The listing builds one solid part. Answer for the finished solid, in the listing's coordinates (mm). A direction names the side the tool comes from. Give positions to 0.01 mm unless a question says otherwise; leave off trailing zeros. Order: outer loops, then holes, each group sorted by start corner. A loop starts at its lowest first (then second) coordinate and runs counter-clockwise, first axis right, second up.
```python
from build123d import *

# Parameters (mm, degrees)
F0_R     = 9.525
F0_R_2   = 5.08
F0_R_3   = 6.35
F0_R_4   = 7.668055
F1_DEPTH = 6.35
F2_DEPTH = 3.175
F3_DEPTH = 12.7


with BuildPart() as f1:
    # F0 (on Front) → F1 (new body, symmetric)
    with BuildSketch(Plane.XZ):
        with BuildLine():
            ThreePointArc((-47.831061, 12.261839), (-40.825144, 16.749128), (-38.1, 24.609932))
            ThreePointArc((-38.1, 24.609932), (-38.532742, 27.896934), (-39.801477, 30.959932))
            ThreePointArc((-39.801477, 30.959932), (-44.45, 35.608455), (-50.8, 37.309932))
            ThreePointArc((-50.8, 37.309932), (-62.469497, 29.621203), (-60.009293, 15.864709))
            ThreePointArc((-60.009293, 15.864709), (-54.40287, 12.4317), (-47.831061, 12.261839))
        make_face()
        with Locations((-50.8, 24.609932)):
            Circle(F0_R, mode=Mode.SUBTRACT)
        with BuildLine():
            ThreePointArc((-50.8, 37.309932), (-44.45, 35.608455), (-39.801477, 30.959932))
            Line((-39.801477, 30.959932), (-6.35, 30.959932))
            ThreePointArc((-6.35, 30.959932), (-4.490128, 35.45006), (0, 37.309932))
            Line((0, 37.309932), (-50.8, 37.309932))
        make_face()
        with BuildLine():
            ThreePointArc((0, 37.309932), (-4.490128, 35.45006), (-6.35, 30.959932))
            ThreePointArc((-6.35, 30.959932), (0, 24.609932), (6.35, 30.959932))
            ThreePointArc((6.35, 30.959932), (4.490128, 35.45006), (0, 37.309932))
        make_face()
        with Locations((0, 30.959932)):
            Circle(F0_R_2, mode=Mode.SUBTRACT)
        with BuildLine():
            Line((50.8, 37.309932), (0, 37.309932))
            ThreePointArc((0, 37.309932), (4.490128, 35.45006), (6.35, 30.959932))
            Line((6.35, 30.959932), (39.801477, 30.959932))
            ThreePointArc((39.801477, 30.959932), (44.45, 35.608455), (50.8, 37.309932))
        make_face()
        with BuildLine():
            ThreePointArc((63.5, 24.609932), (59.780256, 33.590188), (50.8, 37.309932))
            ThreePointArc((50.8, 37.309932), (44.45, 35.608455), (39.801477, 30.959932))
            ThreePointArc((39.801477, 30.959932), (39.130503, 19.598661), (47.831061, 12.261839))
            ThreePointArc((47.831061, 12.261839), (54.40287, 12.4317), (60.009293, 15.864709))
            ThreePointArc((60.009293, 15.864709), (62.595084, 19.901855), (63.5, 24.609932))
        make_face()
        with Locations((50.8, 24.609932)):
            Circle(F0_R_3, mode=Mode.SUBTRACT)
        with BuildLine():
            Line((47.831061, 12.261839), (14.819522, -22.501475))
            ThreePointArc((14.819522, -22.501475), (15.029956, -23.943953), (15.10032, -25.4))
            ThreePointArc((15.10032, -25.4), (14.024374, -30.997911), (10.949864, -35.798084))
            Line((10.949864, -35.798084), (60.009293, 15.864709))
            ThreePointArc((60.009293, 15.864709), (54.40287, 12.4317), (47.831061, 12.261839))
        make_face()
        with BuildLine():
            ThreePointArc((14.819522, -22.501475), (0, -10.29968), (-14.819522, -22.501475))
            ThreePointArc((-14.819522, -22.501475), (-14.498802, -29.619527), (-10.949864, -35.798084))
            ThreePointArc((-10.949864, -35.798084), (0, -40.50032), (10.949864, -35.798084))
            ThreePointArc((10.949864, -35.798084), (14.024374, -30.997911), (15.10032, -25.4))
            ThreePointArc((15.10032, -25.4), (15.029956, -23.943953), (14.819522, -22.501475))
        make_face()
        with Locations((0, -25.4)):
            Circle(F0_R_4, mode=Mode.SUBTRACT)
        with BuildLine():
            Line((-14.819522, -22.501475), (-47.831061, 12.261839))
            ThreePointArc((-47.831061, 12.261839), (-54.40287, 12.4317), (-60.009293, 15.864709))
            Line((-60.009293, 15.864709), (-10.949864, -35.798084))
            ThreePointArc((-10.949864, -35.798084), (-14.498802, -29.619527), (-14.819522, -22.501475))
        make_face()
    extrude(amount=F1_DEPTH, both=True)

    # F0 (on Front) → F2 (join, symmetric)
    with BuildSketch(Plane.XZ):
        with BuildLine():
            ThreePointArc((-39.801477, 30.959932), (-38.532742, 27.896934), (-38.1, 24.609932))
            ThreePointArc((-38.1, 24.609932), (-40.825144, 16.749128), (-47.831061, 12.261839))
            Line((-47.831061, 12.261839), (-14.819522, -22.501475))
            ThreePointArc((-14.819522, -22.501475), (0, -10.29968), (14.819522, -22.501475))
            Line((14.819522, -22.501475), (47.831061, 12.261839))
            ThreePointArc((47.831061, 12.261839), (39.130503, 19.598661), (39.801477, 30.959932))
            Line((39.801477, 30.959932), (6.35, 30.959932))
            ThreePointArc((6.35, 30.959932), (0, 24.609932), (-6.35, 30.959932))
            Line((-6.35, 30.959932), (-39.801477, 30.959932))
        make_face()
    extrude(amount=F2_DEPTH, both=True)

    # F0 (on Front) → F3 (join, symmetric)
    with BuildSketch(Plane.XZ):
        with BuildLine():
            ThreePointArc((63.5, 24.609932), (59.780256, 33.590188), (50.8, 37.309932))
            ThreePointArc((50.8, 37.309932), (44.45, 35.608455), (39.801477, 30.959932))
            ThreePointArc((39.801477, 30.959932), (39.130503, 19.598661), (47.831061, 12.261839))
            ThreePointArc((47.831061, 12.261839), (54.40287, 12.4317), (60.009293, 15.864709))
            ThreePointArc((60.009293, 15.864709), (62.595084, 19.901855), (63.5, 24.609932))
        make_face()
        with Locations((50.8, 24.609932)):
            Circle(F0_R_3, mode=Mode.SUBTRACT)
    extrude(amount=F3_DEPTH, both=True)


solid = f1.part
```
1) For a pull along Z with two mould halves and no side action, classify faces 1 (the cylindrical face through (-46.4, 0.09, 16.16)), 2 (the flat face through (45, 12.7, 28)), 3 (the cylindrical face through (-62.386, -0.089, 29.811)) as +Z half, -Z half, draft (parallel to the pull), parting line (faces both ways), or undercut.
Geometry says:
face 1: undercut
face 2: draft
face 3: parting line
2) Find section C-C (z = -25.4). Write down the section's boundary in (x, y), then the cut area to 3 significant figures.
Geometry says:
outline: (-20.82, -6.35) - (-7.67, -6.35) - (-7.67, 6.35) - (-20.82, 6.35) - close; (7.67, -6.35) - (20.82, -6.35) - (20.82, 6.35) - (7.67, 6.35) - close
area: 334 mm2
3) Find section B-B (z = 21). Write down the section's boundary in (x, y) (3 decimals).
Geometry says:
outline: (-62.976, -6.35) - (-59.614, -6.35) - (-59.614, 6.35) - (-62.976, 6.35) - close; (-41.986, -6.35) - (-38.624, -6.35) - (-38.624, -3.175) - (38.624, -3.175) - (38.624, -12.7) - (45.576, -12.7) - (45.576, 12.7) - (38.624, 12.7) - (38.624, 3.175) - (-38.624, 3.175) - (-38.624, 6.35) - (-41.986, 6.35) - close; (56.024, -12.7) - (62.976, -12.7) - (62.976, 12.7) - (56.024, 12.7) - close
4) Find section A-A (x = 0). Write down the section's boundary in (y, z) (3 decimals).
Geometry says:
outline: (-6.35, -40.5) - (6.35, -40.5) - (6.35, -33.068) - (-6.35, -33.068) - close; (-6.35, -17.732) - (6.35, -17.732) - (6.35, -10.3) - (3.175, -10.3) - (3.175, 24.61) - (6.35, 24.61) - (6.35, 25.88) - (-6.35, 25.88) - (-6.35, 24.61) - (-3.175, 24.61) - (-3.175, -10.3) - (-6.35, -10.3) - close; (-6.35, 36.04) - (6.35, 36.04) - (6.35, 37.31) - (-6.35, 37.31) - close
5) A tool of negligible diameter and unlimited length cuts with its end or side. For faces 4 (the cylindrical face through (-0.661, 0.089, 35.997)), 5 (the flat face through (31.556, -4.785, -4.876)), 6 (the flat face through (-23, 5, 30.96)), from which of +Z, -Z, +X, -X, +Y, -Y can it reach the whole face along a straight path? Write none if from no direction.
Geometry says:
face 4: +Y, -Y
face 5: -Y
face 6: +Y
6) Straight lines are drawn through the part: probe 1 along X at (y, z) = (-5.25, 18); probe 2 along Y at (x, z) = (9, 11) (3 decimals); probe 3 along X at (y, z) = (-3.25, -17.5). For each, find the intervals that lie inside material, in ascending order.
Geometry says:
probe 1: x = -61.64 to -57.66, -43.94 to -39.96, 39.96 to 61.64
probe 2: y = -3.175 to 3.175
probe 3: x = -28.33 to -19.57, -12.87 to 12.87, 19.57 to 28.33
7) Find section D-D (z = -13). Write down the section's boundary in (x, y) (3 decimals), then the cut area to 3 significant figures.
Geometry says:
outline: (-32.599, -6.35) - (-23.842, -6.35) - (-23.842, -3.175) - (-8.617, -3.175) - (-8.617, -6.35) - (8.617, -6.35) - (8.617, -3.175) - (23.842, -3.175) - (23.842, -6.35) - (32.599, -6.35) - (32.599, 6.35) - (23.842, 6.35) - (23.842, 3.175) - (8.617, 3.175) - (8.617, 6.35) - (-8.617, 6.35) - (-8.617, 3.175) - (-23.842, 3.175) - (-23.842, 6.35) - (-32.599, 6.35) - close
area: 635 mm2
8) Given P1, Ø6, axis at y = -0.5, z = -18, coming from the -X side; P2, Ø16, axis at x = 0.5, z = -5, coming from the -Y side; P3, Ø1.6, axis at x = -19.5, y = 5, coming from the -Z side, each flat-ended and moving along its own axis, determine where each tip first touches the part or whether it passes through.
Geometry says:
P1: stops at x = -30.7
P2: stops at y = -6.35
P3: stops at z = -27.64
